Source: CAD feature listing. Evaluate the final solid. Frame: model axes, mm. A direction names the side the tool comes from. Coordinates: 2 decimals unless noted, no trailing zeros. Write each loop counter-clockwise with the first axis right and the second up, starting at its lowest first coordinate (ties: lowest second). Pieces come first, ordered by that corner, then holes. Notation, with made-up numbers: (-0.75, 47.25) - (10.25, 47.25) arc R38 ccw to (10.25, 85.25) - close; hole circle Ø4 at (-33, -9.5). An arc over 180 degrees is marked (long way). One line per question, with ' | ' between items.
from build123d import *

# Parameters (mm, degrees)
F0_R     = 22.5
F1_DEPTH = 5
F2_R     = 1.5
F3_DEPTH = 25
F4_R     = 5
F4_R_2   = 2.3
F5_DEPTH = 1


with BuildPart() as f1:
    # F0 (on Top) → F1 (new body)
    with BuildSketch(Plane.XY):
        Circle(F0_R)
        Polygon((-3.55, -2.049593), (-3.55, 2.049593), (0, 4.099187), (3.55, 2.049593), (3.55, -2.049593), (0, -4.099187), align=None, mode=Mode.SUBTRACT)
    extrude(amount=F1_DEPTH)

    # F2 (on Top) → F3 (cut)
    with BuildSketch(Plane.XY):
        with Locations((-22.5, 0)):
            Circle(F2_R)
        with Locations((-21.665639, -6.070427)):
            Circle(F2_R)
        with Locations((-19.224437, -11.690639)):
            Circle(F2_R)
        with Locations((-15.357446, -16.443809)):
            Circle(F2_R)
        with Locations((-10.351463, -19.977417)):
            Circle(F2_R)
        with Locations((-4.57776, -22.029392)):
            Circle(F2_R)
        with Locations((1.535454, -22.447547)):
            Circle(F2_R)
        with Locations((7.534791, -21.200871)):
            Circle(F2_R)
        with Locations((12.975307, -18.381823)):
            Circle(F2_R)
        with Locations((17.453504, -14.199479)):
            Circle(F2_R)
        with Locations((20.637254, -8.964025)):
            Circle(F2_R)
        with Locations((22.290434, -3.06375)):
            Circle(F2_R)
        with Locations((22.290434, 3.06375)):
            Circle(F2_R)
        with Locations((20.637254, 8.964025)):
            Circle(F2_R)
        with Locations((17.453504, 14.199479)):
            Circle(F2_R)
        with Locations((12.975307, 18.381823)):
            Circle(F2_R)
        with Locations((7.534791, 21.200871)):
            Circle(F2_R)
        with Locations((1.535454, 22.447547)):
            Circle(F2_R)
        with Locations((-4.57776, 22.029392)):
            Circle(F2_R)
        with Locations((-10.351463, 19.977417)):
            Circle(F2_R)
        with Locations((-15.357446, 16.443809)):
            Circle(F2_R)
        with Locations((-19.224437, 11.690639)):
            Circle(F2_R)
        with Locations((-21.665639, 6.070427)):
            Circle(F2_R)
    extrude(amount=F3_DEPTH, mode=Mode.SUBTRACT)

    # F4 (on face) → F5 (join)
    with BuildSketch(Plane.XY.offset(5)):
        Circle(F4_R)
        Circle(F4_R_2, mode=Mode.SUBTRACT)
    extrude(amount=-F5_DEPTH)


solid = f1.part
Item 1: Cut plane C-C on x = -5. Return loops of the section in (y, z).
Check sheet entries:
outline: (-20.59, 0) - (20.59, 0) - (20.59, 5) - (-20.59, 5) - close
Item 2: Cut plane A-A on y = 0. Return loops of the section in (x, z).
Check sheet entries:
outline: (-21, 0) - (-3.55, 0) - (-3.55, 4) - (-2.3, 4) - (-2.3, 5) - (-21, 5) - close; (2.3, 4) - (3.55, 4) - (3.55, 0) - (22.5, 0) - (22.5, 5) - (2.3, 5) - close
Item 3: Ray query, line 1 along Y through (x, z) = (0, 4.65); line 2 along Y through (x, z) = (0, 3.75); line 3 along Y through (x, z) = (6, 3.35). Return the intervals inside material, ascending. Write a range as [from, to].
Check sheet entries:
line 1: [-22.5, -2.3], [2.3, 22.5] | line 2: [-22.5, -4.1], [4.1, 22.5] | line 3: [-21.69, 21.69]
Item 4: Pin query (flat end, axial travel): pin 1 Ø2 at (y, z) = (0, 1.5) entering from -X; pin 2 Ø3.5 at (x, y) = (-1.5, 0) entering from -Z; pin 3 Ø5 at (x, y) = (-10.5, -16.5) entering from -Z; pin 4 Ø3 at (x, y) = (0, 0) entering from -Z. Return the tip coordinate at first contact, or that it passes through.
Check sheet entries:
pin 1: x = -21.38 | pin 2: z = 4 | pin 3: z = 0 | pin 4: through
Item 5: Cut plane B-B on x = -12.5. Return loops of the section in (y, z), and give its area (3 significant figures).
Check sheet entries:
outline: (-18.71, 0) - (18.71, 0) - (18.71, 5) - (-18.71, 5) - close | area: 187 mm²
Item 6: Mould query, pull axis X, two halves, no side actions, for faces 1 (the face through (19.213, -11.709, 2.465)), 2 (the face through (-7.56, -21.19, 2.46)), 3 (the face through (-17.926, -10.939, 2.465)). Classes: pulls with the +X half, pulls with the -X half, needs draft (parallel to the pull), parting line crosses it, or undercut.
Check sheet entries:
face 1: pulls with the +X half | face 2: pulls with the -X half | face 3: undercut
Item 7: Access query for faces 4 (the face through (-1.8, 3.06, 1.97)), 5 (the face through (-21, 0, 2)). Directions: +Z, -Z, +X, -X, +Y, -Y. A direction counts if a zero-diameter tool reaches every point of the face in a straight line with its end or side. Return the directions, or none.
Check sheet entries:
face 4: -Z | face 5: +Z, -Z, -X
